The listing builds one solid part. Answer for the finished solid, in the listing's coordinates (mm). A direction names the side the tool comes from. Round coordinates to 2 decimals unless told otherwise and drop trailing zeros. Loops run counter-clockwise (first coordinate to the right, second up) from the corner with the lowest first, then second, coordinate; pieces in that order, holes last. Notation, with made-up numbers: (76.5, -6) -> (118.5, -6) arc R14 ccw to (118.5, 13) -> close; hole circle Ø11 at (83, 27). An arc over 180 degrees is marked (long way). Use a Markdown table: item, result. Add a question column.
Q1. Section B-B on z = 17.5 is taken. Give the vertices of the cut face in (x, y).
Q2. Which of the six approach directions +Z, -Z, +X, -X, +Y, -Y give full straight-line access (tool end or side, diameter ignored) to faces 1 (the flat face through (-15.423, -1.302, 17.255)), 2 (the cylindrical face through (-4.868, 14.86, 11.151)), 3 (the flat face through (30, 0, 17))?
Q3. For a pull along X with two mould halves and no side action, classify faces 4 (the flat face through (0, 2.5, 17)), 5 (the cylindrical face through (-13.18, 14.86, 14.57)), 6 (the flat face through (-5.8, 25, 23.3)) as released by +X, released by -X, zero draft, split by the parting line, or undercut.
Q4. Given pin 1 Ø6 at (x, y) = (13, 9.5) entering from +Z; pin 2 Ø1 at (x, y) = (5.5, 20.5) entering from +Z; pin 3 Ø1 at (x, y) = (8.5, 15.5) entering from +Z, each flat-ended and moving along its own axis, determine where each tip first touches the part or whether it passes through.
Q5. Consider line 1 (X direction, y = 18, z = 17.5); line 2 (Y direction, x = -25, z = 9); line 3 (X direction, y = 19, z = 22). Determine where each line is inside the solid, lowest interval first.
Q6. Section A-A on x = -19.5 is taken. Give the vertices of the cut face in (y, z), then the cut area to 3 significant figures.
Q7. Section C-C on x = 0 is taken. Give the vertices of the cut face in (y, z), then the cut area to 4 significant figures.
Q8. Section D-D on y = 21 is taken. Give the vertices of the cut face in (x, z).
from build123d import *

# Parameters (mm, degrees)
EXTRUDE_1_DEPTH = 35
SKETCH_2_R      = 13.5
SKETCH_2_R_2    = 8
EXTRUDE_2_DEPTH = 20


with BuildPart() as part:
    # Sketch 1 → Extrude 1 (new body)
    with BuildSketch(Plane.XY):
        Polygon((-30, 5), (-30, -5), (-10, -5), (-21, 2.5), (0, 2.5), (21, 2.5), (10, -5), (30, -5), (30, 5), align=None)
    extrude(amount=EXTRUDE_1_DEPTH)

    # Sketch 2 → Extrude 2 (add)
    with BuildSketch(Plane(origin=(0, 5, 0), x_dir=(1, 0, 0), z_dir=(0, 1, 0))):
        with Locations(Location((0, -17.5, 0), (0, 0, 270))):
            Circle(SKETCH_2_R)
        with Locations(Location((0, -17.5, 0), (0, 0, 270))):
            Circle(SKETCH_2_R_2, mode=Mode.SUBTRACT)
    extrude(amount=EXTRUDE_2_DEPTH)


solid = part.part
Checked values:
| question | item | result |
|---|---|---|
| 1 | outline | (-30, -5) -> (-10, -5) -> (-21, 2.5) -> (21, 2.5) -> (10, -5) -> (30, -5) -> (30, 5) -> (13.5, 5) -> (13.5, 25) -> (8, 25) -> (8, 5) -> (-8, 5) -> (-8, 25) -> (-13.5, 25) -> (-13.5, 5) -> (-30, 5) -> close |
| 2 | face 1 | +Z, -Z |
| 2 | face 2 | +Y |
| 2 | face 3 | +Z, -Z, +X, +Y, -Y |
| 3 | face 4 | undercut |
| 3 | face 5 | split by the parting line |
| 3 | face 6 | zero draft |
| 4 | pin 1 | stops at z = 26.57 |
| 4 | pin 2 | stops at z = 30.04 |
| 4 | pin 3 | stops at z = 28.37 |
| 5 | line 1 | x = -13.5 to -8, 8 to 13.5 |
| 5 | line 2 | y = -5 to 5 |
| 5 | line 3 | x = -12.73 to -6.61, 6.61 to 12.73 |
| 6 | outline | (-5, 0) -> (1.48, 0) -> (1.48, 35) -> (-5, 35) -> close; (2.5, 0) -> (5, 0) -> (5, 35) -> (2.5, 35) -> close |
| 6 | area | 314 mm2 |
| 7 | outline | (2.5, 0) -> (5, 0) -> (5, 4) -> (25, 4) -> (25, 9.5) -> (5, 9.5) -> (5, 25.5) -> (25, 25.5) -> (25, 31) -> (5, 31) -> (5, 35) -> (2.5, 35) -> close |
| 7 | area | 307.5 mm2 |
| 8 | outline | circle Ø27 at (0, 17.5); hole circle Ø16 at (0, 17.5) |
